Source: CAD feature listing. Evaluate the final solid. Frame: model axes, mm. A direction names the side the tool comes from. Round coordinates to 2 decimals unless told otherwise and drop trailing zeros. Write each loop counter-clockwise with the first axis right and the second up, starting at its lowest first coordinate (ties: lowest second). Pieces come first, ordered by that corner, then holes. Notation, with made-up numbers: M 15.5,-33 L 52.5,-33 A11 cw 52.5,-27 Z; hole C 83,32.25 d11. An arc over 180 degrees is marked long. Answer in a Markdown table with one row per item. Add a question column.
Item 1: Material intervals for probe 1 along X at (y, z) = (-75, -371); probe 2 along X at (y, z) = (-11, 100); probe 3 along Y at (x, z) = (51.5, -134), sorted ascending.
Item 2: Mould query, pull axis X, two halves, no side actions, for faces 1 (the face through (56.3, -1.2, -547.3)), 2 (the face through (114.3, -19, -470)), 3 (the face through (109.538, -20, 471)), 4 (the face through (0, 1, 9)). Classes: released by +X, released by -X, zero draft, split by the parting line, or undercut.
Item 3: Cut plane A-A on x = 54. Return loops of the section in (y, z).
Item 4: Cut plane D-D on z = -479. Return loops of the section in (x, y), and give its area (3 significant figures).
Item 5: Set-up query: faces 5 (the face through (56.417, -3.593, -542.957)), 6 (the face through (2, -88.9, 3)). Return all of +Z, -Z, +X, -X, +Y, -Y with unobstructed straight access to the full face (end or side cutting, diameter ignored); none if empty.
Item 6: Contact query for flat-ended pins moving along their axis: pin 1 (10 mm diameter, centred on y = -58, z = 56.5, fed in from +X); pin 2 (5 mm diameter, centred on x = 112.5, y = 15.5, fed in from -Z); pin 3 (5 mm diameter, centred on x = 111, y = -10, fed in from +Z). Output: stop coordinate, or through.
Item 7: Cut plane B-B on z = -142. Return loops of the section in (x, y).
Item 8: Cut plane C-C on y = -31. Return loops of the section in (x, z).
from build123d import *

# Parameters (mm, degrees)
BOSS_EXTRUDE1_DEPTH = 114.3
SHELL3_T            = -4.7625
SKETCH8_W           = 736.6
SKETCH8_H           = 177.8
CUT_EXTRUDE2_DEPTH  = 4.7625


with BuildPart() as part:
    # Sketch1 → Boss-Extrude1 (new body)
    with BuildSketch(Plane(origin=(0, 0, 0), x_dir=(0, 0, -1), z_dir=(1, 0, 0))):
        Polygon((-457.2, 88.9), (-635, -88.9), (-457.2, -88.9), (457.2, -88.9), (635, -88.9), (457.2, 88.9), align=None)
    extrude(amount=BOSS_EXTRUDE1_DEPTH)

    # Shell3
    shell3_openings = [part.faces().sort_by_distance(p)[0] for p in [
        (57.15, -88.9, 0),
    ]]
    offset(amount=SHELL3_T, openings=shell3_openings, kind=Kind.INTERSECTION)

    # Sketch8 → Cut-Extrude2 (cut)
    with BuildSketch(Plane(origin=(114.3, 0, 0), x_dir=(0, 0, -1), z_dir=(1, 0, 0))):
        Rectangle(SKETCH8_W, SKETCH8_H)
    extrude(amount=-CUT_EXTRUDE2_DEPTH, mode=Mode.SUBTRACT)


solid = part.part
Results below:
| question | item | result |
|---|---|---|
| 1 | probe 1 | 0 to 4.76, 109.54 to 114.3 |
| 1 | probe 2 | 0 to 4.76 |
| 1 | probe 3 | 84.14 to 88.9 |
| 2 | face 1 | zero draft |
| 2 | face 2 | released by +X |
| 2 | face 3 | undercut |
| 2 | face 4 | released by -X |
| 3 | outline | M -88.9,-635 L 88.9,-457.2 L 88.9,457.2 L -88.9,635 L -88.9,628.26 L 84.14,455.23 L 84.14,-455.23 L -88.9,-628.26 Z |
| 4 | outline | M 0,-88.9 L 4.76,-88.9 L 4.76,60.36 L 109.54,60.36 L 109.54,-88.9 L 114.3,-88.9 L 114.3,67.1 L 0,67.1 Z |
| 4 | area | 2,190 mm2 |
| 5 | face 5 | -Y |
| 5 | face 6 | +Z, -Z, +X, -X, -Y |
| 6 | pin 1 | x = 4.76 |
| 6 | pin 2 | z = -533.1 |
| 6 | pin 3 | z = 558.6 |
| 7 | outline | M 0,-88.9 L 4.76,-88.9 L 4.76,84.14 L 109.54,84.14 L 109.54,88.9 L 0,88.9 Z |
| 8 | outline | M 0,-577.1 L 114.3,-577.1 L 114.3,-368.3 L 109.54,-368.3 L 109.54,-570.36 L 4.76,-570.36 L 4.76,570.36 L 109.54,570.36 L 109.54,368.3 L 114.3,368.3 L 114.3,577.1 L 0,577.1 Z |
